```python
from build123d import *

# Parameters (mm, degrees)
SKETCH1_W          = 165.1
SKETCH1_H          = 22.225
BASE_EXTRUDE_DEPTH = 8.89
SKETCH3_W          = 158.75
SKETCH3_H          = 12.5095
PIECE_CUT_DEPTH    = 6.35
CORNER_CUT_DEPTH   = 167.826235122


with BuildPart() as part:
    # Sketch1 → Base Extrude (new body)
    with BuildSketch(Plane(origin=(0, 0, 0), x_dir=(1, 0, 0), z_dir=(0, 1, 0))):
        with Locations((82.55, 11.1125)):
            Rectangle(SKETCH1_W, SKETCH1_H)
    extrude(amount=BASE_EXTRUDE_DEPTH)

    # Sketch3 → Piece Cut (cut)
    with BuildSketch(Plane(origin=(0, 8.89, 0), x_dir=(1, 0, 0), z_dir=(0, 1, 0))):
        with Locations((82.55, 11.1125)):
            Rectangle(SKETCH3_W, SKETCH3_H)
    extrude(amount=-PIECE_CUT_DEPTH, mode=Mode.SUBTRACT)

    # Sketch4 → Corner Cut (cut, through all)
    with BuildSketch(Plane(origin=(0, 0, -22.225), x_dir=(-1, 0, 0), z_dir=(0, 0, -1))):
        Polygon((0, 0), (-8.89, 8.89), (0, 8.89), align=None)
        Polygon((-165.1, 8.89), (-156.21, 8.89), (-165.1, 0), align=None)
    extrude(amount=-CORNER_CUT_DEPTH, mode=Mode.SUBTRACT)


solid = part.part
```
Source: CAD feature listing. Evaluate the final solid. Frame: model axes, mm. Round coordinates to 2 decimals unless told otherwise and drop trailing zeros. Loops run counter-clockwise (first coordinate to the right, second up) from the corner with the lowest first, then second, coordinate; pieces in that order, holes last.
1. Section query A-A on y = 5.25. Output: boundary loops of the cut face in (x, z) (3 decimals), and give its area (3 significant figures).
2. Section query C-C on z = -15. Output: boundary loops of the cut face in (x, y) (3 decimals), and give its area (3 significant figures).
3. Mould query, pull axis X, two halves, no side actions, for faces 1 (the flat face through (82, 8.89, -2)), 2 (the flat face through (81, 2.54, -11)), 3 (the flat face through (162.6, 2.5, -11.3)). Classes: released by +X, released by -X, zero draft, split by the parting line, or undercut.
4. Ray query, L1, parallel to Z at x = 25, y = 7.75 (3 decimals); L2, parallel to Y at x = 96, z = -12; L3, parallel to X at y = 1, z = -17. Return the intervals inside material, ascending.
5. Section query B-B on x = 50. Output: boundary loops of the cut face in (y, z) (3 decimals).
6. Contact query for flat-ended pins moving along their axis: pin 1 (5 mm diameter, centred on x = 146, z = -13.5, fed in from +Y); pin 2 (0.5 mm diameter, centred on y = 3, z = -12, fed in from -X); pin 3 (0.7 mm diameter, centred on y = 3, z = -8, fed in from +X). Output: stop coordinate, or through.
Answers below:
1. outline: (5.25, -22.225) - (159.85, -22.225) - (159.85, -17.367) - (5.25, -17.367) - close; (5.25, -4.858) - (159.85, -4.858) - (159.85, 0) - (5.25, 0) - close
1. area: 1,500 mm2
2. outline: (0, 0) - (165.1, 0) - (161.925, 3.175) - (161.925, 2.54) - (3.175, 2.54) - (3.175, 3.175) - close
2. area: 413 mm2
3. face 1: zero draft
3. face 2: undercut
3. face 3: released by +X
4. L1: z = -22.225 to -17.367, -4.858 to 0
4. L2: y = 0 to 2.54
4. L3: x = 1 to 164.1
5. outline: (0, -22.225) - (8.89, -22.225) - (8.89, -17.367) - (2.54, -17.367) - (2.54, -4.858) - (8.89, -4.858) - (8.89, 0) - (0, 0) - close
6. pin 1: stops at y = 2.54
6. pin 2: stops at x = 2.75
6. pin 3: stops at x = 162.45
